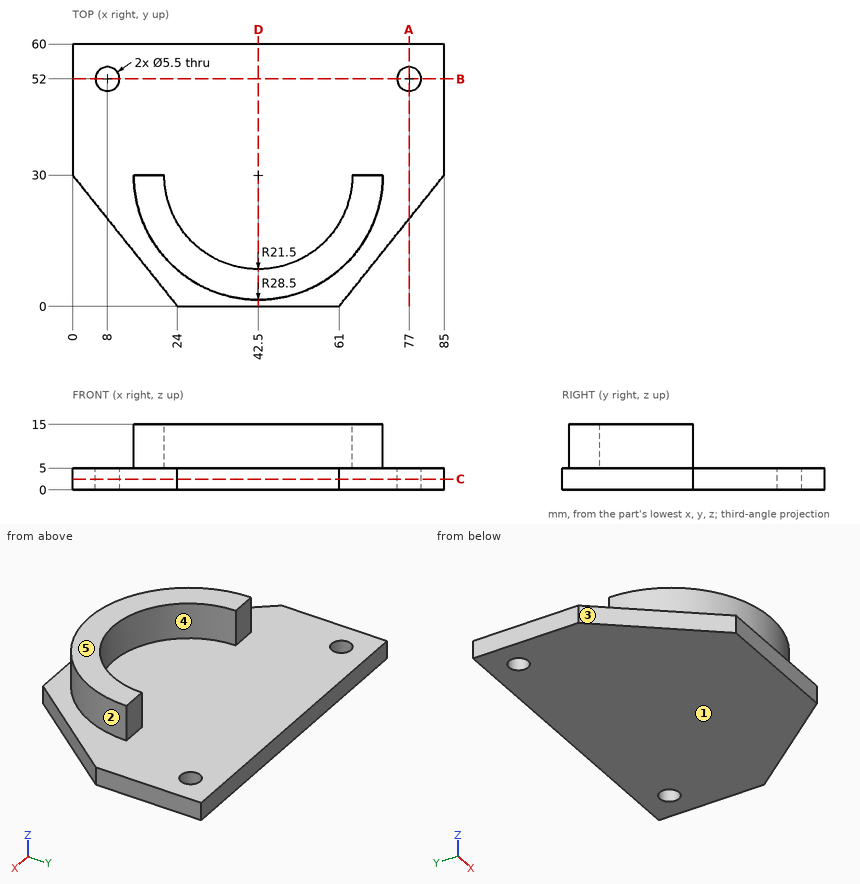
Job drawing, mm, ordinate dimensions from the low corner. One solid piece. A direction names the side the tool comes from. Coordinates: 2 decimals unless noted, no trailing zeros. Loops run counter-clockwise (first coordinate to the right, second up) from the corner with the lowest first, then second, coordinate; pieces in that order, holes last. Notation, with made-up numbers: (-11.75, -22) - (32.25, -22) arc R9 cw to (32.25, -5) - close; hole circle Ø11 at (30, -37.75). An arc over 180 degrees is marked (long way). Answer as a JSON object with one key per item and string values. Group by question number.
(1) Cut at D-D (x = 42.5). Give the cut face in (y, z), then the cut area to 3 significant figures.
(2) Flat gauge pins, fed straight in: pin 1 (1.5 mm diameter, centred on x = 67.5, y = 48.5, fed in from +Z); pin 2 (7.5 mm diameter, centred on x = 17, z = 10.5, fed in from +Y); pin 3 (8 mm diameter, centred on y = 13.5, z = 7, fed in from +X). Where does each tip first touch, or does it go through?
(3) Cut at A-A (x = 77). Give the cut face in (y, z).
(4) Cut at B-B (y = 52). Give the cut face in (x, z).
(5) Probe line 1 along X through (y, z) = (52, 3.5); line 2 along Z through (x, y) = (60, 45.5); line 3 along X through (y, z) = (10.5, 7). List the from-to ranges inside material, lowest first.
(6) Tool access for the marked faces 1 and 2: list every direction of +Z, -Z, +X, -X, +Y, -Y with a clear straight run to the whole face (end or side of a thin tool).
(7) Cut at C-C (z = 2.5). Give the cut face in (x, y).
(8) Two-plate mould, pull along X, no slides. Class the marked faces 3, 4 and 5: released by +X, released by -X, zero draft, split by the parting line, or undercut.
Geometry says:
{
 "1": {"outline": "(0, 0) - (60, 0) - (60, 5) - (8.5, 5) - (8.5, 15) - (1.5, 15) - (1.5, 5) - (0, 5) - close", "area": "370 mm^2"},
 "2": {"pin 1": "stops at z = 5", "pin 2": "stops at y = 30", "pin 3": "stops at x = 74.57"},
 "3": {"outline": "(20, 0) - (49.25, 0) - (49.25, 5) - (20, 5) - close; (54.75, 0) - (60, 0) - (60, 5) - (54.75, 5) - close"},
 "4": {"outline": "(0, 0) - (5.25, 0) - (5.25, 5) - (0, 5) - close; (10.75, 0) - (74.25, 0) - (74.25, 5) - (10.75, 5) - close; (79.75, 0) - (85, 0) - (85, 5) - (79.75, 5) - close"},
 "5": {"line 1": "x = 0 to 5.25, 10.75 to 74.25, 79.75 to 85", "line 2": "z = 0 to 5", "line 3": "x = 21.72 to 33.44, 51.56 to 63.28"},
 "6": {"face 1": "-Z, +X, -X, +Y, -Y", "face 2": "+Z, -Y"},
 "7": {"outline": "(0, 30) - (24, 0) - (61, 0) - (85, 30) - (85, 60) - (0, 60) - close; hole circle Ø5.5 at (8, 52); hole circle Ø5.5 at (77, 52)"},
 "8": {"face 3": "released by -X", "face 4": "undercut", "face 5": "zero draft"}
}
